The listing builds one solid part. Answer for the finished solid, in the listing's coordinates (mm). Give positions to 0.01 mm unless a question says otherwise; leave off trailing zeros. Write each loop counter-clockwise with the first axis right and the second up, starting at its lowest first coordinate (ties: lowest second). Pieces come first, ordered by that corner, then holes. Notation, with made-up numbers: (83, 74.25) -> (130, 74.25) arc R14 cw to (130, 97.25) -> close; hole circle Ø3 at (4, 30.5). An arc over 180 degrees is marked (long way). Put each result on its own line as item: value. Start each with the question number.
1) A cutting plane is placed at A-A (z = -214). Write down the section's boundary in (x, y), then the cut area to 3 significant figures.
2) A cutting plane is placed at C-C (x = 1.5). Write down the section's boundary in (y, z) (1 decimal).
3) A cutting plane is placed at B-B (y = 112.5). Write down the section's boundary in (x, z).
4) A cutting plane is placed at D-D (z = -267). Write down the section's boundary in (x, y).
5) Flat-ended cylindrical pins translate along their axes: pin 1 Ø3 at (x, z) = (5.5, -258.5) entering from -Y; pin 2 Ø7.5 at (y, z) = (147.03, -272.76) entering from +X; pin 3 Ø2 at (x, z) = (1, -270) entering from -Y; pin 4 Ø3 at (y, z) = (106.05, -296.11) entering from -X. Find the tip coordinate at first contact, or state that the pin passes through.
6) Find the intervals of material crossed by line 1 along Z through (x, y) = (1, 181); line 2 along Y through (x, z) = (1.5, -271); line 3 along Y through (x, z) = (1.5, -285), in increasing order. Write a range as from..to.
from build123d import *

# Parameters (mm, degrees)
SKETCH1_R           = 2.6289
SKETCH1_R_2         = 14.2875
SKETCH1_R_3         = 3.2639
BOSS_EXTRUDE1_DEPTH = 6.35
FILLET1_R           = 4.7625


with BuildPart() as part:
    # Sketch1 → Boss-Extrude1 (new body)
    with BuildSketch(Plane(origin=(0, 0, 0), x_dir=(0, 0, -1), z_dir=(1, 0, 0))):
        with BuildLine():
            Line((261.600661049, 84.883471899), (235.704081281, 147.403346332))
            Line((235.704081281, 147.403346332), (204.461245323, 156.764386521))
            ThreePointArc((204.461245323, 156.764386521), (189.925416447, 179.241173024), (209.807662792, 197.163018154))
            Line((209.807662792, 197.163018154), (241.790461139, 198.057364052))
            Line((241.790461139, 198.057364052), (272.292637552, 198.910306814))
            ThreePointArc((272.292637552, 198.910306814), (291.249324985, 187.666425791), (289.242335043, 165.717556793))
            Line((289.242335043, 165.717556793), (282.117070677, 156.43173152))
            Line((282.117070677, 156.43173152), (304.408641761, 102.615117992))
            Line((304.408641761, 102.615117992), (261.600661049, 84.883471899))
        make_face()
        with Locations((296.111966941, 106.051713243)):
            Circle(SKETCH1_R, mode=Mode.SUBTRACT)
        with Locations((249.178886841, 125.492031649)):
            Circle(SKETCH1_R, mode=Mode.SUBTRACT)
        with Locations((272.645426891, 115.771872446)):
            Circle(SKETCH1_R_2, mode=Mode.SUBTRACT)
        with Locations((210.384530747, 176.533582155)):
            Circle(SKETCH1_R_2, mode=Mode.SUBTRACT)
        with Locations((272.869505507, 178.280870816)):
            Circle(SKETCH1_R_2, mode=Mode.SUBTRACT)
        with Locations((272.757466199, 147.026371631)):
            Circle(SKETCH1_R_3, mode=Mode.SUBTRACT)
        with Locations((244.504033835, 151.048406008)):
            Circle(SKETCH1_R_3, mode=Mode.SUBTRACT)
    extrude(amount=BOSS_EXTRUDE1_DEPTH)

    # Fillet1
    fillet1_edges = [part.edges().sort_by_distance(p)[0] for p in [
        (3.175, 156.43173152, -282.117070677),
    ]]
    fillet(fillet1_edges, radius=FILLET1_R)


solid = part.part
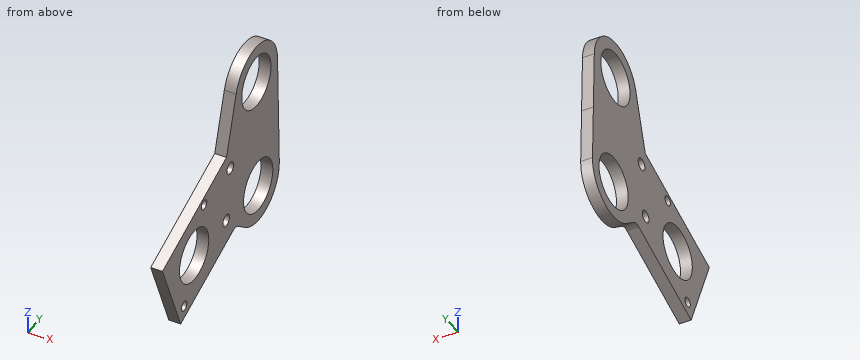
Reply:
1. outline: (0, 153.91) -> (6.35, 153.91) -> (6.35, 162.71) -> (0, 162.71) -> close; (0, 190.36) -> (6.35, 190.36) -> (6.35, 197.28) -> (0, 197.28) -> close
1. area: 99.9 mm2
2. outline: (84.9, -261.6) -> (102.6, -304.4) -> (153.9, -283.2) arc R4.8 cw to (158.6, -283.8) -> (165.7, -289.2) arc R20.6 ccw to (198.9, -272.3) -> (197.2, -209.8) arc R20.6 ccw to (156.8, -204.5) -> (147.4, -235.7) -> close; hole circle Ø28.6 at (115.8, -272.6); hole circle Ø5.3 at (106.1, -296.1); hole circle Ø5.3 at (125.5, -249.2); hole circle Ø6.5 at (147, -272.8); hole circle Ø6.5 at (151, -244.5); hole circle Ø28.6 at (176.5, -210.4); hole circle Ø28.6 at (178.3, -272.9)
3. outline: (0, -300.31) -> (6.35, -300.31) -> (6.35, -286.55) -> (0, -286.55) -> close; (0, -258.74) -> (6.35, -258.74) -> (6.35, -250.16) -> (0, -250.16) -> close
4. outline: (0, 87.12) -> (6.35, 87.12) -> (6.35, 102.65) -> (0, 102.65) -> close; (0, 128.9) -> (6.35, 128.9) -> (6.35, 165.25) -> (0, 165.25) -> close; (0, 191.31) -> (6.35, 191.31) -> (6.35, 198.76) -> (0, 198.76) -> close
5. pin 1: stops at y = 88.75
5. pin 2: stops at x = 6.35
5. pin 3: stops at y = 87.95
5. pin 4: passes through
6. line 1: z = -293.33..-286.9, -258.84..-223.96, -196.81..-190.24
6. line 2: y = 88.78..101.58, 129.96..144.28, 149.78..164.12, 192.45..198.87
6. line 3: y = 94.58..108.6, 122.95..149.47, 160.19..170.73, 185.83..194.98
